Geometry: final body of the model. Coordinates: model frame, mm. Face numbers are marked on the shaded views. A direction names the side the tool comes from. Round coordinates to 2 decimals unless told otherwise and drop trailing zeros. Order: outer loops, then holes, each group sorted by start corner. A loop starts at its lowest first (then second) coordinate and runs counter-clockwise, first axis right, second up. Notation, with made-up numbers: M -30.75,61 L -22.75,61 A22 cw -22.75,81 Z; hole C -26,84 d3. An arc over 180 degrees is marked long. Put each result on its own line as item: value. Start each with the question number.
1) Access query for the marked faces 1, 2, 3, 4 and 5. Directions: +Z, -Z, +X, -X, +Y, -Y. A direction counts if a zero-diameter tool reaches every point of the face in a straight line with its end or side. Return the directions, or none.
2) Material intervals for probe 1 along X at (y, z) = (9.5, -1.5); probe 2 along X at (y, z) = (-16, -0.5); probe 3 along Y at (x, z) = (-25, 0.75), sorted ascending. Write a range as [from, to].
3) Draft query along Y for the marked faces 6, 7, 8 and 9. Return one class per face: pulls with the +Y half, pulls with the -Y half, needs draft (parallel to the pull), parting line crosses it, or undercut.
4) Section A-A, the plane y = 11. Return loops of the section in (x, z) (3 decimals).
5) Section D-D, the plane z = 0.75. Return loops of the section in (x, y).
6) Section C-C, the plane y = -16.5. Return loops of the section in (x, z) (3 decimals).
7) First-contact query: P1, Ø3, axis at y = -4, z = -1.5, coming from the -X side; P2, Ø2, axis at x = 5.5, y = -14.5, coming from the -Z side (3 decimals). Flat tips, straight axial feed; report the tip coordinate or a pass-through.
8) Section B-B, the plane x = -26. Return loops of the section in (y, z) (3 decimals).
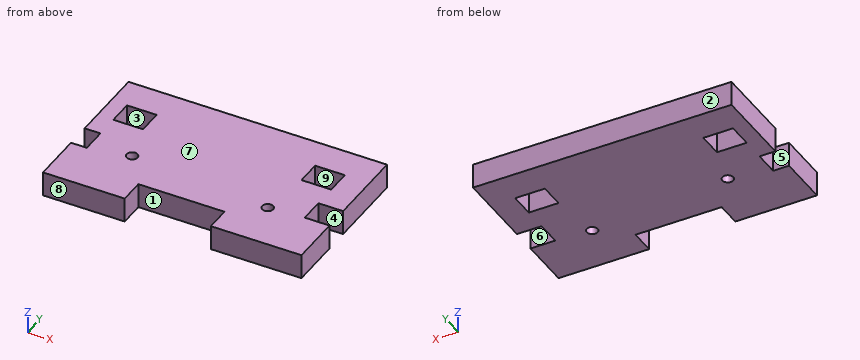
from build123d import *

# Parameters (mm, degrees)
SKETCH1_W             = 66.294
SKETCH1_H             = 39.878
BOSS_EXTRUDE1_DEPTH   = 3.175
CAVITY1_START         = -19.939
CAVITY1_OUTLINE_W     = 22.098
CAVITY1_OUTLINE_H     = 6.35
CAVITY1_DEPTH         = 6.35
CAVITY1_START_2       = 5.461
CAVITY1_2_OUTLINE_W   = 7.62
CAVITY1_2_OUTLINE_H   = 6.35
CAVITY1_2_DEPTH       = 6.35
CAVITY1_START_3       = -6.879912323
CAVITY1_3_OUTLINE_W   = 6.35
CAVITY1_3_OUTLINE_H   = 6.35
CAVITY1_3_OUTLINE_W_2 = 4.064
CAVITY1_3_DEPTH       = 6.35
SKETCH4_R             = 1.397
CUT_EXTRUDE1_DEPTH    = 40.199615177


# Read off the part's stored shape, not the designer's step: Cavity1
with BuildPart() as part:
    # Sketch1 → Boss-Extrude1 (new, symmetric)
    with BuildSketch(Plane.XY):
        Rectangle(SKETCH1_W, SKETCH1_H)
    extrude(amount=BOSS_EXTRUDE1_DEPTH, both=True)

    # Cavity1 outline → Cavity1 (cut)
    with BuildSketch(Plane(origin=(0, 0, 0), x_dir=(1, 0, 0), z_dir=(0, 1, 0)).offset(CAVITY1_START)):
        with Locations((-1.143, 0)):
            Rectangle(CAVITY1_OUTLINE_W, CAVITY1_OUTLINE_H)
    extrude(amount=CAVITY1_DEPTH, mode=Mode.SUBTRACT)

    # Cavity1 2 outline → Cavity1 2 (cut)
    with BuildSketch(Plane(origin=(0, 0, 0), x_dir=(1, 0, 0), z_dir=(0, 1, 0)).offset(CAVITY1_START_2)):
        with Locations((22.987, 0)):
            Rectangle(CAVITY1_2_OUTLINE_W, CAVITY1_2_OUTLINE_H)
        with Locations((-25.273, 0)):
            Rectangle(CAVITY1_2_OUTLINE_W, CAVITY1_2_OUTLINE_H)
    extrude(amount=CAVITY1_2_DEPTH, mode=Mode.SUBTRACT)

    # Cavity1 3 outline → Cavity1 3 (cut)
    with BuildSketch(Plane(origin=(0, 0, 0), x_dir=(1, 0, 0), z_dir=(0, 1, 0)).offset(CAVITY1_START_3)):
        with Locations((29.972, 0)):
            Rectangle(CAVITY1_3_OUTLINE_W, CAVITY1_3_OUTLINE_H)
        with Locations((-31.115, 0)):
            Rectangle(CAVITY1_3_OUTLINE_W_2, CAVITY1_3_OUTLINE_H)
    extrude(amount=CAVITY1_3_DEPTH, mode=Mode.SUBTRACT)

    # Sketch4 → Cut-Extrude1 (cut, through all)
    with BuildSketch(Plane(origin=(0, 0, -3.175), x_dir=(-1, 0, 0), z_dir=(0, 0, -1))):
        with Locations((-17.653, -7.493)):
            Circle(SKETCH4_R)
        with Locations((18.669, -4.699)):
            Circle(SKETCH4_R)
    extrude(amount=-CUT_EXTRUDE1_DEPTH, mode=Mode.SUBTRACT)


solid = part.part
Result sheet:
1. face 1: +Z, -Z, -Y
1. face 2: +Z, -Z, +X, -X, +Y
1. face 3: +Z, -Z
1. face 4: +Z, -Z, +X
1. face 5: +Z, -Z, -X
2. probe 1: x = [-33.15, -29.08], [-21.46, 19.18], [26.8, 33.15]
2. probe 2: x = [-33.15, -12.19], [9.91, 33.15]
2. probe 3: y = [-19.94, 5.46], [11.81, 19.94]
3. face 6: undercut
3. face 7: needs draft
3. face 8: pulls with the -Y half
3. face 9: undercut
4. outline: M -33.147,-3.175 L -29.083,-3.175 L -29.083,3.175 L -33.147,3.175 Z; M -21.463,-3.175 L 19.177,-3.175 L 19.177,3.175 L -21.463,3.175 Z; M 26.797,-3.175 L 33.147,-3.175 L 33.147,3.175 L 26.797,3.175 Z
5. outline: M -33.15,-19.94 L -12.19,-19.94 L -12.19,-13.59 L 9.91,-13.59 L 9.91,-19.94 L 33.15,-19.94 L 33.15,-6.88 L 26.8,-6.88 L 26.8,-0.53 L 33.15,-0.53 L 33.15,19.94 L -33.15,19.94 L -33.15,-0.53 L -29.08,-0.53 L -29.08,-6.88 L -33.15,-6.88 Z; hole M -29.08,5.46 L -21.46,5.46 L -21.46,11.81 L -29.08,11.81 Z; hole C -18.67,-4.7 d2.79; hole C 17.65,-7.49 d2.79; hole M 19.18,5.46 L 26.8,5.46 L 26.8,11.81 L 19.18,11.81 Z
6. outline: M -33.147,-3.175 L -12.192,-3.175 L -12.192,3.175 L -33.147,3.175 Z; M 9.906,-3.175 L 33.147,-3.175 L 33.147,3.175 L 9.906,3.175 Z
7. P1: stops at x = -29.08
7. P2: stops at z = -3.175
8. outline: M -19.939,-3.175 L 5.461,-3.175 L 5.461,3.175 L -19.939,3.175 Z; M 11.811,-3.175 L 19.939,-3.175 L 19.939,3.175 L 11.811,3.175 Z
